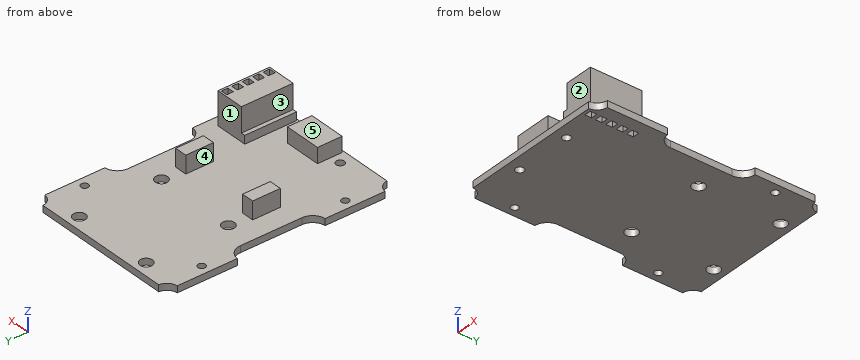
from build123d import *

# Parameters (mm, degrees)
EXTRUDE_1_DEPTH     = 1.6
SKETCH_2_3_R        = 0.9
SKETCH_2_3_W        = 1.6
SKETCH_2_3_H        = 1.6
CUT_EXTRUDE_4_DEPTH = 35.167821119
SKETCH_3_W          = 9
SKETCH_3_H          = 6
EXTRUDE_2_DEPTH     = 3.7
SKETCH_4_R          = 1.5
CUT_EXTRUDE_5_DEPTH = 35.33030731
SKETCH_8_W          = 8
SKETCH_8_H          = 12.6
SKETCH_8_W_2        = 1.6
SKETCH_8_H_2        = 1.6
EXTRUDE_7_DEPTH     = 8
SKETCH_9_W          = 3
SKETCH_9_H          = 6.75
EXTRUDE_9_DEPTH     = 4.3
SKETCH_10_R         = 1
CUT_EXTRUDE_6_DEPTH = 36.05538475
SKETCH_11_W         = 1
SKETCH_11_H         = 6
CUT_EXTRUDE_7_DEPTH = 12.6


with BuildPart() as part:
    # 草图2 → 凸台-拉伸1 (new body)
    with BuildSketch(Plane.XY):
        with BuildLine():
            Line((19.8, 10.693743885), (19.8, 25.307417596))
            ThreePointArc((19.8, 25.307417596), (18.090811691, 26.090811691), (17.307417596, 27.8))
            Line((17.307417596, 27.8), (-17.307417596, 27.8))
            ThreePointArc((-17.307417596, 27.8), (-18.090811691, 26.090811691), (-19.8, 25.307417596))
            Line((-19.8, 25.307417596), (-19.8, 10.693743885))
            ThreePointArc((-19.8, 10.693743885), (-17.667619242, 9.69089023), (-16.8, 7.5))
            Line((-16.8, 7.5), (-16.8, -7.5))
            ThreePointArc((-16.8, -7.5), (-17.667619242, -9.69089023), (-19.8, -10.693743885))
            Line((-19.8, -10.693743885), (-19.8, -25.307417596))
            ThreePointArc((-19.8, -25.307417596), (-18.090811691, -26.090811691), (-17.307417596, -27.8))
            Line((-17.307417596, -27.8), (17.307417596, -27.8))
            ThreePointArc((17.307417596, -27.8), (18.090811691, -26.090811691), (19.8, -25.307417596))
            Line((19.8, -25.307417596), (19.8, -10.693743885))
            ThreePointArc((19.8, -10.693743885), (17.667619242, -9.69089023), (16.8, -7.5))
            Line((16.8, -7.5), (16.8, 7.5))
            ThreePointArc((16.8, 7.5), (17.667619242, 9.69089023), (19.8, 10.693743885))
        make_face()
    extrude(amount=EXTRUDE_1_DEPTH)

    # 草图2<3> → 切除-拉伸4 (cut, through all)
    with BuildSketch(Plane.XY):
        with Locations((17.5, 17.5)):
            Circle(SKETCH_2_3_R)
        with Locations((-17.5, 17.5)):
            Circle(SKETCH_2_3_R)
        with Locations((-17.5, -17.5)):
            Circle(SKETCH_2_3_R)
        with Locations((16, -16.04)):
            Rectangle(SKETCH_2_3_W, SKETCH_2_3_H)
        with Locations((16, -18.58)):
            Rectangle(SKETCH_2_3_W, SKETCH_2_3_H)
        with Locations((16, -21.12)):
            Rectangle(SKETCH_2_3_W, SKETCH_2_3_H)
        with Locations((16, -23.66)):
            Rectangle(SKETCH_2_3_W, SKETCH_2_3_H)
        with Locations((16, -26.2)):
            Rectangle(SKETCH_2_3_W, SKETCH_2_3_H)
    extrude(amount=CUT_EXTRUDE_4_DEPTH, mode=Mode.SUBTRACT)

    # 草图3 → 凸台-拉伸2 (add)
    with BuildSketch(Plane.XY.offset(1.6)):
        with Locations((0, -24.3)):
            Rectangle(SKETCH_3_W, SKETCH_3_H)
    extrude(amount=EXTRUDE_2_DEPTH)

    # 草图4 → 切除-拉伸5 (cut, through all)
    with BuildSketch(Plane.XY.offset(1.6)):
        with Locations((-10, 24.9)):
            Circle(SKETCH_4_R)
        with Locations((10, 24.9)):
            Circle(SKETCH_4_R)
        with Locations((-10, 4.9)):
            Circle(SKETCH_4_R)
        with Locations((10, 4.9)):
            Circle(SKETCH_4_R)
    extrude(amount=-CUT_EXTRUDE_5_DEPTH, mode=Mode.SUBTRACT)

    # 草图8 → 凸台-拉伸7 (add)
    with BuildSketch(Plane.XY.offset(1.6)):
        with Locations((13.3, -21.12)):
            Rectangle(SKETCH_8_W, SKETCH_8_H)
        with Locations((16, -26.2)):
            Rectangle(SKETCH_8_W_2, SKETCH_8_H_2, mode=Mode.SUBTRACT)
        with Locations((16, -23.66)):
            Rectangle(SKETCH_8_W_2, SKETCH_8_H_2, mode=Mode.SUBTRACT)
        with Locations((16, -21.12)):
            Rectangle(SKETCH_8_W_2, SKETCH_8_H_2, mode=Mode.SUBTRACT)
        with Locations((16, -18.58)):
            Rectangle(SKETCH_8_W_2, SKETCH_8_H_2, mode=Mode.SUBTRACT)
        with Locations((16, -16.04)):
            Rectangle(SKETCH_8_W_2, SKETCH_8_H_2, mode=Mode.SUBTRACT)
    extrude(amount=EXTRUDE_7_DEPTH)

    # 草图9 → 凸台-拉伸9 (add)
    with BuildSketch(Plane.XY.offset(1.6)):
        with Locations((-10, -3.175)):
            Rectangle(SKETCH_9_W, SKETCH_9_H)
        with Locations((10, -3.175)):
            Rectangle(SKETCH_9_W, SKETCH_9_H)
    extrude(amount=EXTRUDE_9_DEPTH)

    # 草图10 → 切除-拉伸6 (cut, through all)
    with BuildSketch(Plane.XY.offset(1.6)):
        with Locations((-7, -24.8)):
            Circle(SKETCH_10_R)
        with Locations(Location((7, -24.8, 0), (0, 0, 180))):
            Circle(SKETCH_10_R)
    extrude(amount=-CUT_EXTRUDE_6_DEPTH, mode=Mode.SUBTRACT)

    # 草图11 → 切除-拉伸7 (cut)
    with BuildSketch(Plane.XZ.offset(27.42)):
        with Locations((9.8, 6.6)):
            Rectangle(SKETCH_11_W, SKETCH_11_H)
    extrude(amount=-CUT_EXTRUDE_7_DEPTH, mode=Mode.SUBTRACT)


solid = part.part
The model under review builds one solid part; all positions refer to its coordinate system, in mm. Face numbers are marked on the shaded views. A direction names the side the tool comes from. Round coordinates to 2 decimals unless told otherwise and drop trailing zeros. Loops run counter-clockwise (first coordinate to the right, second up) from the corner with the lowest first, then second, coordinate; pieces in that order, holes last. Notation, with made-up numbers: (40, -22) -> (79, -22) arc R21 ccw to (79, -16) -> close; hole circle Ø9 at (-33.75, 57.5). An arc over 180 degrees is marked (long way). Answer as CSV lines item,"result".
1) Add section B-B on x = -10. Write out the cut boundary in (y, z).
Geometry results:
outline,"(-27.8, 0) -> (3.4, 0) -> (3.4, 1.6) -> (0.2, 1.6) -> (0.2, 5.9) -> (-6.55, 5.9) -> (-6.55, 1.6) -> (-27.8, 1.6) -> close; (6.4, 0) -> (23.4, 0) -> (23.4, 1.6) -> (6.4, 1.6) -> close; (26.4, 0) -> (27.8, 0) -> (27.8, 1.6) -> (26.4, 1.6) -> close"
2) To check wall thickness, follow line 1 along X through (y, z) = (0, 5.75); line 2 along Z through (x, y) = (14, -4.5); line 3 along Y through (x, z) = (7, 0.3). State the ranges of each line that lie inside material, in increasing order. Write a range as from..to.
Geometry results:
line 1,"x = -11.5..-8.5, 8.5..11.5"
line 2,"z = 0..1.6"
line 3,"y = -27.8..-25.8, -23.8..27.8"
3) Tool access review of the marked faces 1, 2, 3, 4 and 5: name each direction out of +Z, -Z, +X, -X, +Y, -Y from which nothing blocks a thin tool from reaching the whole face with its end or side.
Geometry results:
face 1,"+Z, +X, -X"
face 2,"+Z, +X, -X, -Y"
face 3,"+Z, -Y"
face 4,"+Z, +Y, -Y"
face 5,"+Z, -X, +Y, -Y"
4) For P1, Ø1.8, axis at x = 16.5, z = 3.5, coming from the +Y side; P2, Ø6.5, axis at x = 2, y = -23.5, coming from the +Z side; P3, Ø1.3, axis at y = -2, z = 4, coming from the -X side, all flat-tipped, find the tip position at first contact; note any pin that passes through.
Geometry results:
P1,"stops at y = -14.82"
P2,"stops at z = 5.3"
P3,"stops at x = -11.5"
5) Add section C-C on z = 2.5. State how many separate pieces and enclosed holes the cut face has, plus the area to 4 significant figures.
Geometry results:
separate pieces,"4"
enclosed holes,"5"
area,"182.5 mm²"
6) Add section D-D on x = -1. Write out the cut boundary in (y, z), plus the area to 3 significant figures.
Geometry results:
outline,"(-27.8, 0) -> (27.8, 0) -> (27.8, 1.6) -> (-21.3, 1.6) -> (-21.3, 5.3) -> (-27.3, 5.3) -> (-27.3, 1.6) -> (-27.8, 1.6) -> close"
area,"111 mm²"
7) Add section A-A on y = 4.9. Write out the cut boundary in (x, z), plus the area to 3 significant figures.
Geometry results:
outline,"(-16.8, 0) -> (-11.5, 0) -> (-11.5, 1.6) -> (-16.8, 1.6) -> close; (-8.5, 0) -> (8.5, 0) -> (8.5, 1.6) -> (-8.5, 1.6) -> close; (11.5, 0) -> (16.8, 0) -> (16.8, 1.6) -> (11.5, 1.6) -> close"
area,"44.2 mm²"
